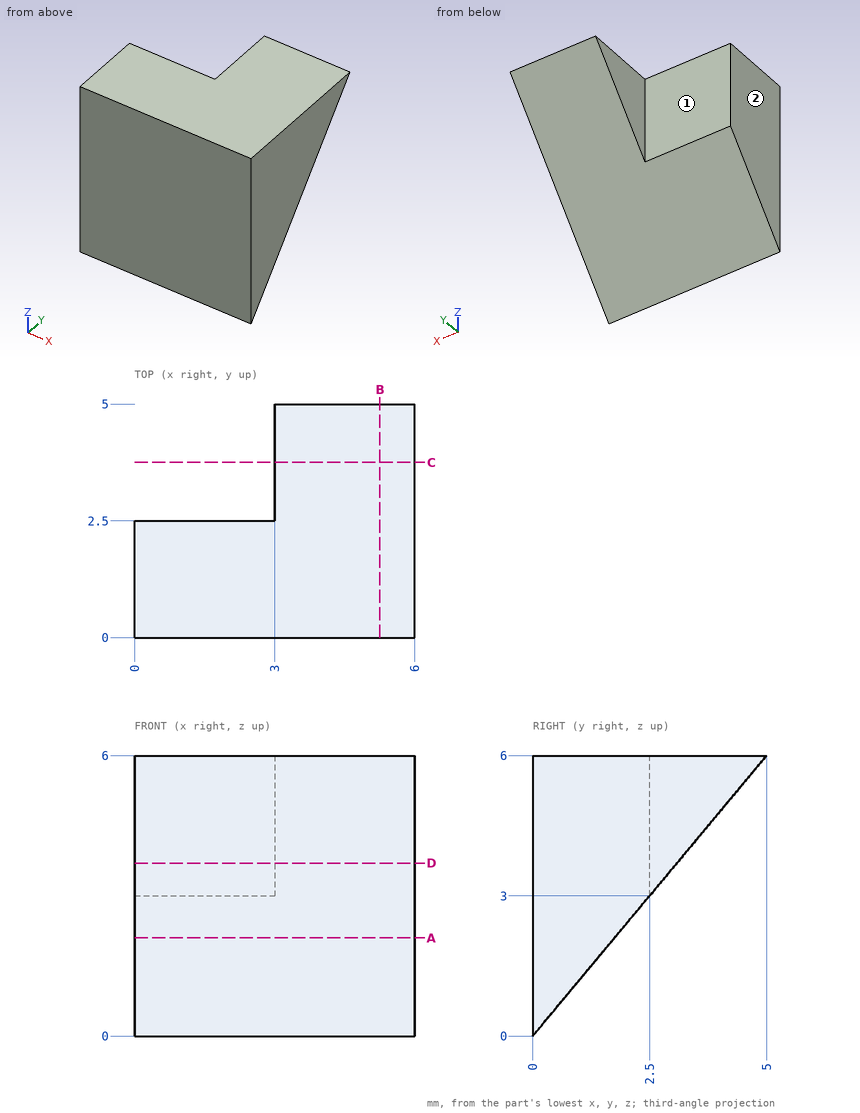
Job drawing, mm, ordinate dimensions from the low corner. One solid piece. A direction names the side the tool comes from. Coordinates: 2 decimals unless noted, no trailing zeros. Write each loop counter-clockwise with the first axis right and the second up, starting at its lowest first coordinate (ties: lowest second). Pieces come first, ordered by that corner, then holes. Notation, with made-up numbers: (-6.75, 50) -> (40.25, 50) arc R13 cw to (40.25, 62) -> close; hole circle Ø8 at (-28, 31.25). An arc over 180 degrees is marked (long way). Use CSV: the item, a comma, the result in double quotes. Start each with the question number.
Item 1: Band-saw the part on D-D, the plane z = 3.7. Write the cut outline in (x, y).
Item 2: Band-saw the part on A-A, the plane z = 2.1. Write the cut outline in (x, y).
Item 3: Tool access for the marked faces 1 and 2: list every direction of +Z, -Z, +X, -X, +Y, -Y with a clear straight run to the whole face (end or side of a thin tool).
Item 4: Drop flat-ended pins along their axis: P1, Ø0.8, axis at y = 4, z = 4, coming from the -X side (3 decimals); P2, Ø1.5, axis at x = 3.5, z = 3.5, coming from the +Y side; P3, Ø1, axis at x = 0.5, z = 3.5, coming from the +Y side; P4, Ø3.5, axis at x = 2, z = 4, coming from the +Y side. Give the stop position or say it passes through.
Item 5: Wall check: probe 1 along X at (y, z) = (4.25, 5.15); probe 2 along Y at (x, z) = (1.7, 3.7); probe 3 along Y at (x, z) = (1.85, 2.15). Give the ranges that are in metal, low to high.
Item 6: Band-saw the part on B-B, the plane x = 5.25. Write the cut outline in (y, z).
Item 7: Band-saw the part on C-C, the plane y = 3.75. Write the cut outline in (x, z), plus the area to 3 significant figures.
Response values:
1,outline,"(0, 0) -> (6, 0) -> (6, 3.08) -> (3, 3.08) -> (3, 2.5) -> (0, 2.5) -> close"
2,outline,"(0, 0) -> (6, 0) -> (6, 1.75) -> (0, 1.75) -> close"
3,face 1,"+Z, -Z, -X, +Y"
3,face 2,"+Z, -Z, -X, +Y, -Y"
4,P1,"passes through"
4,P2,"stops at y = 3.54"
4,P3,"stops at y = 2.5"
4,P4,"stops at y = 4.53"
5,probe 1,"x = 3 to 6"
5,probe 2,"y = 0 to 2.5"
5,probe 3,"y = 0 to 1.79"
6,outline,"(0, 0) -> (5, 6) -> (0, 6) -> close"
7,outline,"(3, 4.5) -> (6, 4.5) -> (6, 6) -> (3, 6) -> close"
7,area,"4.50 mm2"
